Work out the finished part from the listing and answer in its coordinate system (mm). Face numbers are marked on the shaded views. A direction names the side the tool comes from. Coordinates: 2 decimals unless noted, no trailing zeros. Order: outer loops, then holes, each group sorted by start corner. A loop starts at its lowest first (then second) coordinate and runs counter-clockwise, first axis right, second up. Notation, with made-up numbers: (5.25, -18) - (21.25, -18) arc R25 ccw to (21.25, 21) - close; hole circle Ø11 at (19.5, 44.5). An arc over 180 degrees is marked (long way). Answer as a JSON object with one key per item and string values. Group by question number.
1) Section C-C (z = 6.25) is taken. Give the vertices of the cut face in (x, y), plus the area to 3 significant figures.
2) Find the intervals of material crossed by line 1 along Y through (x, z) = (1.5, -7.75); line 2 along Z through (x, y) = (-4.5, -4.75); line 3 along Z through (x, y) = (-14.5, -8.25), in increasing order.
3) Section B-B (x = 7) is taken. Give the vertices of the cut face in (y, z).
4) The mould has two halves that part along X. Classify the marked faces 4 and 5: released by +X, released by -X, zero draft, split by the parting line, or undercut.
5) A tool of negligible diameter and unlimited length cuts with its end or side. For the marked faces 1, 2 and 3, from which of +Z, -Z, +X, -X, +Y, -Y can it reach the whole face along a straight path? Write none if from no direction.
6) Section D-D (y = -10.25) is taken. Give the vertices of the cut face in (x, z).
7) Section A-A (z = 0) is taken. Give the vertices of the cut face in (x, y), plus the area to 3 significant figures.
8) Each of these flat-tipped pins is pushed along its axis until it touches: P1, Ø3, axis at y = -6, z = -7.5, coming from the +X side; P2, Ø0.8, axis at y = -6.5, z = 6, coming from the -X side; P3, Ø1.1, axis at x = -3, y = -2, coming from the +Z side. Where does it stop, or does it pass through?
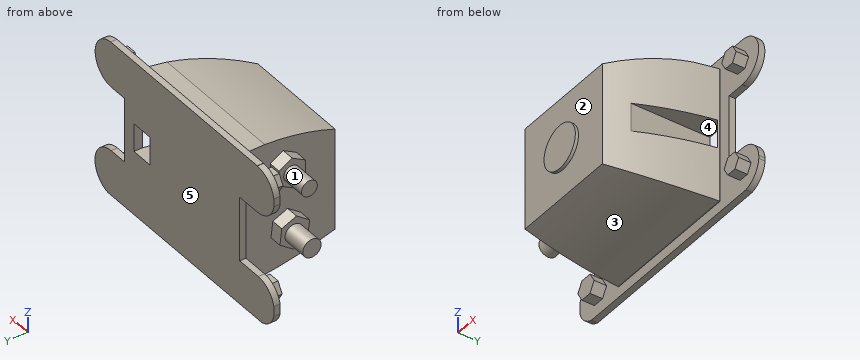
from build123d import *

# Parameters (mm, degrees)
SKETCH2_W            = 40
SKETCH2_H            = 25
BOSS_EXTRUDE2_DEPTH  = 1
CUT_EXTRUDE1_DEPTH   = 24.606143268
SKETCH5_W            = 3.048166118
SKETCH5_H            = 10.380355358
CUT_EXTRUDE4_DEPTH   = 1
CUT_EXTRUDE5_DEPTH   = 24.606143268
SKETCH7_W            = 4.145565418
SKETCH7_H            = 10.399948371
CUT_EXTRUDE7_DEPTH   = 24.606143268
SKETCH8_W            = 22.680519054
SKETCH8_H            = 21.612113122
BOSS_EXTRUDE3_DEPTH  = 15
CUT_EXTRUDE8_DEPTH   = 30
CUT_EXTRUDE9_DEPTH   = 30
CUT_EXTRUDE10_DEPTH  = 30
SKETCH12_W           = 3.628157273
SKETCH12_H           = 4.536406583
CUT_EXTRUDE11_DEPTH  = 29.500000056
BOSS_EXTRUDE4_DEPTH  = 2
BOSS_EXTRUDE5_DEPTH  = 2
BOSS_EXTRUDE6_DEPTH  = 2
BOSS_EXTRUDE7_DEPTH  = 2
SKETCH17_R           = 3.503719222
BOSS_EXTRUDE8_DEPTH  = 0.5
BOSS_EXTRUDE9_DEPTH  = 2
BOSS_EXTRUDE10_DEPTH = 2
SKETCH20_R           = 1.26687785
BOSS_EXTRUDE11_DEPTH = 4
SKETCH21_R           = 1.46158904
BOSS_EXTRUDE12_DEPTH = 4


with BuildPart() as part:
    # Sketch2 → Boss-Extrude2 (new body)
    with BuildSketch(Plane(origin=(0, 0, 0), x_dir=(1, 0, 0), z_dir=(0, 1, 0))):
        Rectangle(SKETCH2_W, SKETCH2_H)
    extrude(amount=BOSS_EXTRUDE2_DEPTH)

    # Sketch4 → Cut-Extrude1 (cut, through all)
    with BuildSketch(Plane(origin=(0, 0, 0), x_dir=(-1, 0, 0), z_dir=(0, -1, 0))):
        with BuildLine():
            Line((-16.311436799, -5.195321305), (-16.311436799, 5.197856111))
            ThreePointArc((-16.311436799, 5.197856111), (-20.005849228, 9.049958295), (-16.002782134, 12.580231412))
            Line((-16.002782134, 12.580231412), (-16.034433084, 14.57463247))
            Line((-16.034433084, 14.57463247), (-22.167227524, 14.47730562))
            Line((-22.167227524, 14.47730562), (-21.947479334, -14.537250164))
            Line((-21.947479334, -14.537250164), (-16.200353352, -14.798286616))
            Line((-16.200353352, -14.798286616), (-16.311436799, -12.504458481))
            ThreePointArc((-16.311436799, -12.504458481), (-19.966005387, -8.849889893), (-16.311436799, -5.195321305))
        make_face()
    extrude(amount=-CUT_EXTRUDE1_DEPTH, mode=Mode.SUBTRACT)

    # Sketch5 → Cut-Extrude4 (cut)
    with BuildSketch(Plane(origin=(0, 0, 0), x_dir=(-1, 0, 0), z_dir=(0, -1, 0))):
        with Locations((-14.87035518, 0.008277846)):
            Rectangle(SKETCH5_W, SKETCH5_H)
    extrude(amount=-CUT_EXTRUDE4_DEPTH, mode=Mode.SUBTRACT)

    # Sketch6 → Cut-Extrude5 (cut, through all)
    with BuildSketch(Plane(origin=(0, 0, 0), x_dir=(-1, 0, 0), z_dir=(0, -1, 0))):
        with BuildLine():
            Line((16.521680561, 5.46762026), (16.29742638, -4.945125741))
            ThreePointArc((16.29742638, -4.945125741), (20.054665472, -8.702364833), (16.29742638, -12.459603925))
            Line((16.29742638, -12.459603925), (16.29742638, -15.143532095))
            Line((16.29742638, -15.143532095), (29.009035652, -15.661685945))
            Line((29.009035652, -15.661685945), (29.009035652, -13.80156801))
            Line((29.009035652, -13.80156801), (27.951962111, 14.649001906))
            Line((27.951962111, 14.649001906), (18.760629252, 18.072251543))
            Line((18.760629252, 18.072251543), (16.723599762, 12.602882354))
            ThreePointArc((16.723599762, 12.602882354), (20.090739839, 8.937108322), (16.521680561, 5.46762026))
        make_face()
    extrude(amount=-CUT_EXTRUDE5_DEPTH, mode=Mode.SUBTRACT)

    # Sketch7 → Cut-Extrude7 (cut, through all)
    with BuildSketch(Plane(origin=(0, 0, 0), x_dir=(-1, 0, 0), z_dir=(0, -1, 0))):
        with Locations((14.448897852, 0.267646074)):
            Rectangle(SKETCH7_W, SKETCH7_H)
    extrude(amount=-CUT_EXTRUDE7_DEPTH, mode=Mode.SUBTRACT)

    # Sketch8 → Boss-Extrude3 (add)
    with BuildSketch(Plane(origin=(0, 0, 0), x_dir=(-1, 0, 0), z_dir=(0, -1, 0))):
        Rectangle(SKETCH8_W, SKETCH8_H)
    extrude(amount=BOSS_EXTRUDE3_DEPTH)

    # Sketch9 → Cut-Extrude8 (cut)
    with BuildSketch(Plane(origin=(0, 0, -10.806056561), x_dir=(-1, 0, 0), z_dir=(0, 0, -1))):
        with BuildLine():
            Line((-11.340259527, -15), (-5.948771171, -15))
            ThreePointArc((-5.948771171, -15), (-9.260644908, -7.752061524), (-11.340259527, -0.059446699))
            Line((-11.340259527, -0.059446699), (-11.340259527, -15))
        make_face()
    extrude(amount=-CUT_EXTRUDE8_DEPTH, mode=Mode.SUBTRACT)

    # Sketch10 → Cut-Extrude9 (cut)
    with BuildSketch(Plane.ZY.offset(11.340259527)):
        with BuildLine():
            Line((-10.806056561, -15), (-7.993035408, -15))
            ThreePointArc((-7.993035408, -15), (-9.83110735, -7.639316506), (-10.806056561, -0.115511352))
            Line((-10.806056561, -0.115511352), (-10.806056561, -15))
        make_face()
    extrude(amount=-CUT_EXTRUDE9_DEPTH, mode=Mode.SUBTRACT)

    # Sketch11 → Cut-Extrude10 (cut)
    with BuildSketch(Plane.ZY.offset(11.340259527)):
        with BuildLine():
            ThreePointArc((10.806056561, -3.748163783), (10.041226218, -9.472321419), (8.369186868, -15))
            Line((8.369186868, -15), (10.806056561, -15))
            Line((10.806056561, -15), (10.806056561, -3.748163783))
        make_face()
    extrude(amount=-CUT_EXTRUDE10_DEPTH, mode=Mode.SUBTRACT)

    # Sketch12 → Cut-Extrude11 (cut, through all)
    with BuildSketch(Plane(origin=(0, 1, 0), x_dir=(1, 0, 0), z_dir=(0, 1, 0))):
        with Locations((9.470946216, -0.081192325)):
            Rectangle(SKETCH12_W, SKETCH12_H)
    extrude(amount=-CUT_EXTRUDE11_DEPTH, mode=Mode.SUBTRACT)

    # Sketch13 → Boss-Extrude4 (add)
    with BuildSketch(Plane(origin=(0, 0, 0), x_dir=(-1, 0, 0), z_dir=(0, -1, 0))):
        Polygon((-14.494931401, -8.884648292), (-15.301061446, -7.488390096), (-16.913321537, -7.488390096), (-17.719451582, -8.884648292), (-16.913321537, -10.280906489), (-15.301061446, -10.280906489), align=None)
    extrude(amount=BOSS_EXTRUDE4_DEPTH)

    # Sketch14 → Boss-Extrude5 (add)
    with BuildSketch(Plane(origin=(0, 0, 0), x_dir=(-1, 0, 0), z_dir=(0, -1, 0))):
        Polygon((-15.042408021, 8.784141367), (-15.850363425, 10.183561177), (-17.466274234, 10.183561177), (-18.274229638, 8.784141367), (-17.466274234, 7.384721557), (-15.850363425, 7.384721557), align=None)
    extrude(amount=BOSS_EXTRUDE5_DEPTH)

    # Sketch15 → Boss-Extrude6 (add)
    with BuildSketch(Plane(origin=(0, 0, 0), x_dir=(-1, 0, 0), z_dir=(0, -1, 0))):
        Polygon((17.871524181, -8.889197459), (17.023921653, -7.421106816), (15.328716596, -7.421106816), (14.481114068, -8.889197459), (15.328716596, -10.357288103), (17.023921653, -10.357288103), align=None)
    extrude(amount=BOSS_EXTRUDE6_DEPTH)

    # Sketch16 → Boss-Extrude7 (add)
    with BuildSketch(Plane(origin=(0, 0, 0), x_dir=(-1, 0, 0), z_dir=(0, -1, 0))):
        Polygon((17.673273489, 8.94154839), (16.76404939, 10.516370724), (14.945601192, 10.516370724), (14.036377093, 8.94154839), (14.945601192, 7.366726055), (16.76404939, 7.366726055), align=None)
    extrude(amount=BOSS_EXTRUDE7_DEPTH)

    # Sketch17 → Boss-Extrude8 (add)
    with BuildSketch(Plane(origin=(0, -15, 0), x_dir=(-1, 0, 0), z_dir=(0, -1, 0))):
        with Locations(Location((2.881571025, 0, 0), (0, 0, 90))):
            Circle(SKETCH17_R)
    extrude(amount=BOSS_EXTRUDE8_DEPTH)

    # Sketch18 → Boss-Extrude9 (add)
    with BuildSketch(Plane.ZY.offset(11.340259527)):
        Polygon((3.659390597, -6.726148666), (4.869302964, -8.821778359), (7.2891277, -8.821778359), (8.499040067, -6.726148666), (7.2891277, -4.630518972), (4.869302964, -4.630518972), align=None)
    extrude(amount=BOSS_EXTRUDE9_DEPTH)

    # Sketch19 → Boss-Extrude10 (add)
    with BuildSketch(Plane.ZY.offset(11.340259527)):
        Polygon((-6.402752553, -6.836831629), (-5.363301958, -9.210722079), (-2.787727224, -9.497476683), (-1.251603086, -7.410340836), (-2.291053681, -5.036450385), (-4.866628415, -4.749695782), align=None)
    extrude(amount=BOSS_EXTRUDE10_DEPTH)

    # Sketch20 → Boss-Extrude11 (add)
    with BuildSketch(Plane.ZY.offset(13.340259527)):
        with Locations((6.055236467, -6.614121956)):
            Circle(SKETCH20_R)
    extrude(amount=BOSS_EXTRUDE11_DEPTH)

    # Sketch21 → Boss-Extrude12 (add)
    with BuildSketch(Plane.ZY.offset(13.340259527)):
        with Locations((-3.88229524, -7.020150319)):
            Circle(SKETCH21_R)
    extrude(amount=BOSS_EXTRUDE12_DEPTH)


solid = part.part
Report:
{
 "1": {"outline": "(-19.14, 0) - (-11.34, 0) - (-11.34, -4.63) - (-13.34, -4.63) - (-13.34, -5.36) - (-17.34, -5.36) - (-17.34, -7.87) - (-13.34, -7.87) - (-13.34, -8.82) - (-11.34, -8.82) - (-11.34, -15) - (5.95, -15) arc R48.47 ccw to (11.34, -0.06) - (11.34, 0) - (18.88, 0) - (18.88, 1) - (-19.14, 1) - close", "area": "363 mm²"},
 "2": {"line 1": "y = -15 to 1", "line 2": "z = -10.31 to 10.74", "line 3": "z = -4.67 to -3.09"},
 "3": {"outline": "(-13.02, -8.58) arc R65.53 ccw to (-0.12, -10.81) - (0, -10.81) - (0, -12.5) - (1, -12.5) - (1, 12.5) - (0, 12.5) - (0, 10.81) - (-3.75, 10.81) arc R35.93 ccw to (-13.02, 9.08) - close"},
 "4": {"face 4": "undercut", "face 5": "zero draft"},
 "5": {"face 1": "-X", "face 2": "-Y", "face 3": "-Z, +X, -X, -Y"},
 "6": {"outline": "(-11.34, -9.28) - (8.28, -9.28) - (8.28, -2.19) - (7.66, -2.19) - (7.66, 2.35) - (8.28, 2.35) - (8.28, 9.86) - (-11.34, 9.86) - close"},
 "7": {"outline": "(-12.38, 0) - (-11.34, 0) - (-11.34, -15) - (-6.39, -15) - (-6.39, -15.5) - (0.62, -15.5) - (0.62, -15) - (5.95, -15) arc R48.47 ccw to (7.66, -11.66) - (7.66, 1) - (-12.38, 1) - close; (11.29, -0.35) arc R48.47 ccw to (11.34, -0.06) - (11.34, 0) - (13.35, 0) - (13.35, 1) - (11.29, 1) - close", "area": "308 mm²"},
 "8": {"P1": "stops at x = 10.31", "P2": "stops at x = -17.34", "P3": "stops at z = 10.81"}
}
